Answer from the drawing. Dimensions are ordinates in mm from the lowest x, y and z of the part. A direction names the side the tool comes from. Give positions to 0.01 mm unless a question says otherwise; leave off trailing zeros. Loops run counter-clockwise (first coordinate to the right, second up) from the corner with the lowest first, then second, coordinate; pieces in that order, holes last. Notation, with made-up numbers: (-28, -5.5) - (18, -5.5) arc R20 cw to (18, 0.5) - close; hole circle Ø1 at (31, 14). An arc over 180 degrees is marked (long way). One line per item, written item: value.
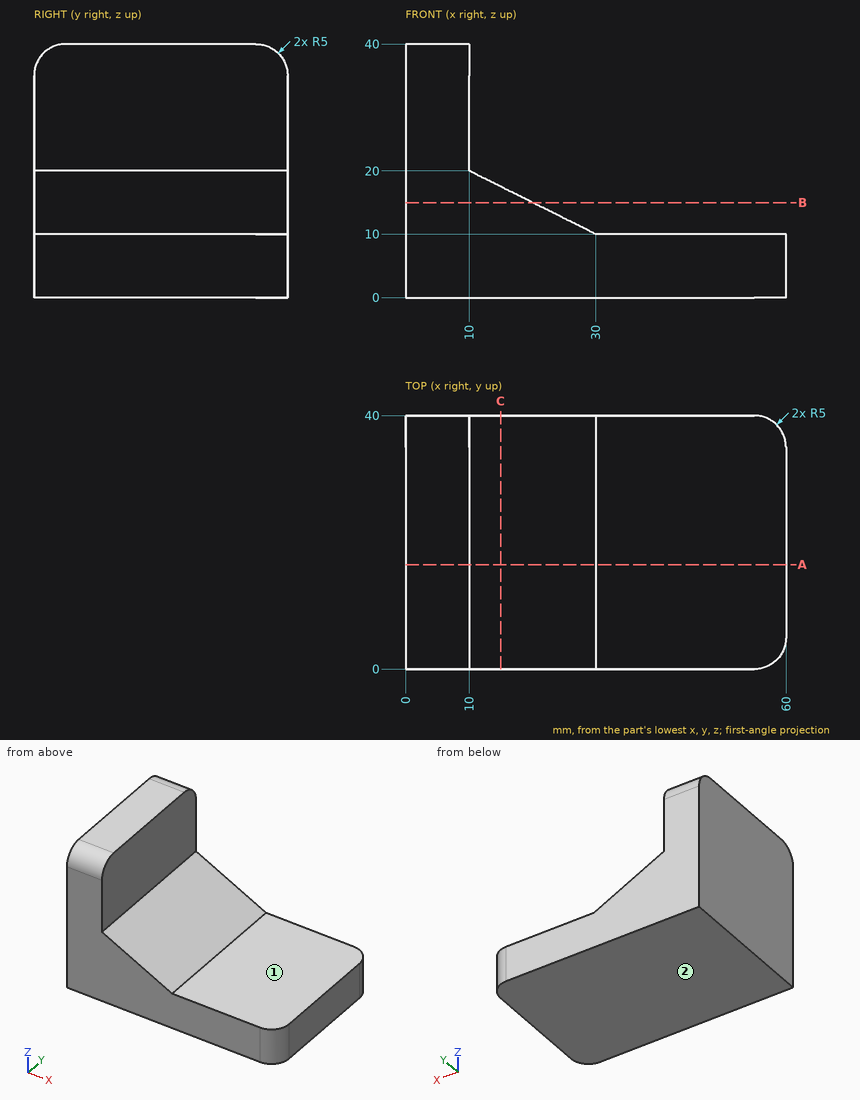
1. Flat-ended cylindrical pins translate along their axes: pin 1 Ø4 at (x, y) = (31, 14) entering from +Z; pin 2 Ø6 at (x, z) = (25.5, 17.5) entering from -Y; pin 3 Ø6 at (y, z) = (9, 34.5) entering from +X; pin 4 Ø12 at (x, y) = (52, 13) entering from +Z. Find the tip coordinate at first contact, or state that the pin passes through.
Output:
pin 1: stops at z = 10.5
pin 2: passes through
pin 3: stops at x = 10
pin 4: stops at z = 10
2. Section A-A (y = 16.5) is taken. Write down the section's boundary in (x, z), and give its area (3 significant figures).
Output:
outline: (0, 0) - (60, 0) - (60, 10) - (30, 10) - (10, 20) - (10, 40) - (0, 40) - close
area: 1,000 mm²
3. For the marked faces 1 and 2, determine the directions among +Z, -Z, +X, -X, +Y, -Y from which every point of the face is accessible in a straight line to the end or side of a thin tool.
Output:
face 1: +Z, +X, +Y, -Y
face 2: -Z, +X, -X, +Y, -Y
4. Section B-B (z = 15) is taken. Write down the section's boundary in (x, y).
Output:
outline: (0, 0) - (20, 0) - (20, 40) - (0, 40) - close
5. Section C-C (x = 15) is taken. Write down the section's boundary in (y, z), and give its area (3 significant figures).
Output:
outline: (0, 0) - (40, 0) - (40, 17.5) - (0, 17.5) - close
area: 700 mm²
6. Find the intervals of material crossed by line 1 along Z through (x, y) = (46, 29); line 2 along X through (y, z) = (25, 16.5), in increasing order.
Output:
line 1: z = 0 to 10
line 2: x = 0 to 17
